The drawing under review shows one solid part. Ordinate dimensions are in mm from its lowest x, y, z. A direction names the side the tool comes from. Give positions to 0.01 mm unless a question says otherwise; leave off trailing zeros. Order: outer loops, then holes, each group sorted by start corner. A loop starts at its lowest first (then second) coordinate and runs counter-clockwise, first axis right, second up. Notation, with made-up numbers: (-34, 19) - (-16, 19) arc R19 ccw to (-16, 41) - close; hole circle Ø2 at (83.5, 17). An arc over 180 degrees is marked (long way). Use CSV: the item, a comma, the result in double quotes.
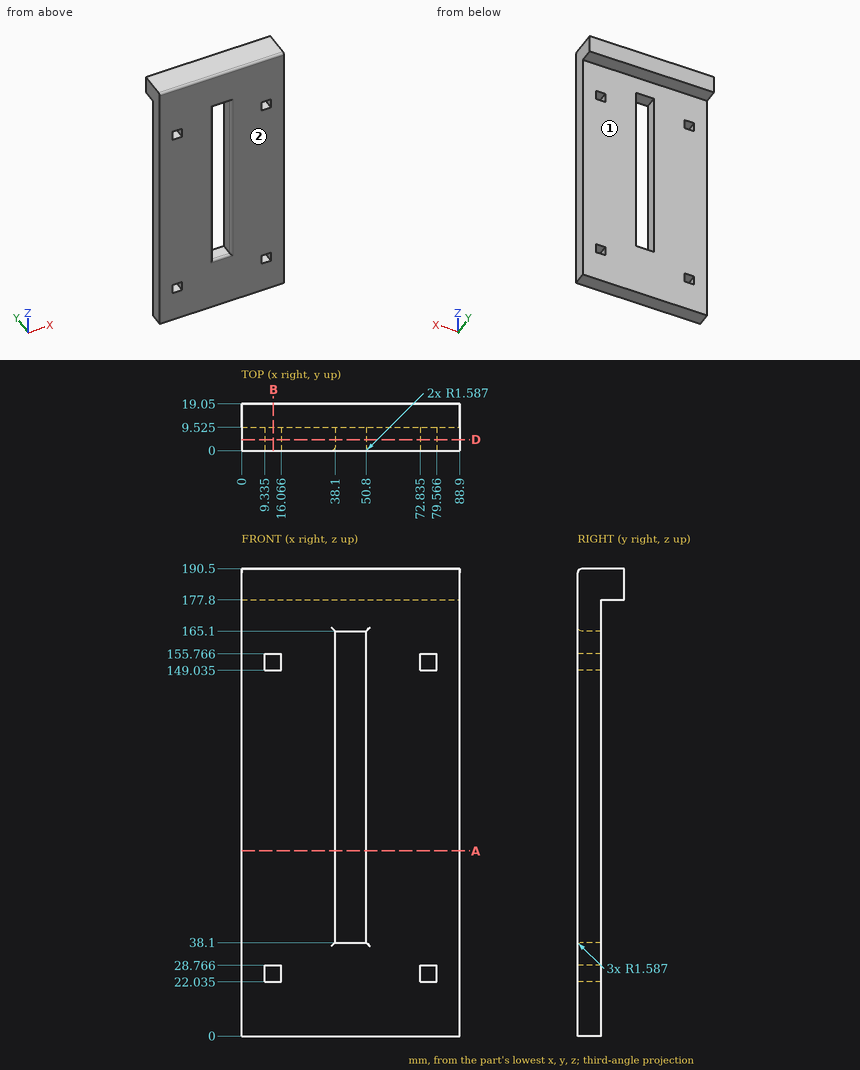
Item 1: Take a section at D-D, the plane y = 4.5. Give the boundary of the cut face in (x, z) (1 decimal).
Results list:
outline,"(0, 0) - (88.9, 0) - (88.9, 190.5) - (0, 190.5) - close; hole (9.3, 22) - (16.1, 22) - (16.1, 28.8) - (9.3, 28.8) - close; hole (9.3, 149) - (16.1, 149) - (16.1, 155.8) - (9.3, 155.8) - close; hole (38.1, 38.1) - (50.8, 38.1) - (50.8, 165.1) - (38.1, 165.1) - close; hole (72.8, 22) - (79.6, 22) - (79.6, 28.8) - (72.8, 28.8) - close; hole (72.8, 149) - (79.6, 149) - (79.6, 155.8) - (72.8, 155.8) - close"
Item 2: Tool access review of the marked faces 1 and 2: name each direction out of +Z, -Z, +X, -X, +Y, -Y from which nothing blocks a thin tool from reaching the whole face with its end or side.
Results list:
face 1,"-Z, +X, -X, +Y"
face 2,"+Z, -Z, +X, -X, -Y"
Item 3: Take a section at A-A, the plane z = 75.5. Give the boundary of the cut face in (x, y) (1 decimal), and give its area (3 significant figures).
Results list:
outline,"(0, 0) - (36.5, 0) arc R1.6 ccw to (38.1, 1.6) - (38.1, 9.5) - (0, 9.5) - close; (50.8, 1.6) arc R1.6 ccw to (52.4, 0) - (88.9, 0) - (88.9, 9.5) - (50.8, 9.5) - close"
area,"725 mm2"
Item 4: Take a section at B-B, the plane x = 13. State how many separate pieces and enclosed holes the cut face has, and give its area (3 significant figures).
Results list:
separate pieces,"3"
enclosed holes,"0"
area,"1,810 mm2"
Item 5: Wall thickness on L1, parallel to X at y = 9, z = 27.5 (1 decimal); L2, parallel to X at y = 5.5, z = 145.5; L3, parallel to Z at x = 47.5, y = 4.25: over which ranges is each line inside the solid? List them lowest first.
Results list:
L1,"x = 0 to 9.3, 16.1 to 72.8, 79.6 to 88.9"
L2,"x = 0 to 38.1, 50.8 to 88.9"
L3,"z = 0 to 38.1, 165.1 to 190.5"
Item 6: Clearance check with flat-ended pins moving along their axes: pin 1 (5 mm diameter, centred on x = 61, z = 36, fed in from +Y) (1 decimal); pin 2 (6 mm diameter, centred on x = 31, y = 15, fed in from -Z). State where each tip first meets the part, or that it passes through.
Results list:
pin 1,"stops at y = 9.5"
pin 2,"stops at z = 177.8"
